Here's how the part is built. I have some questions about the finished solid (model axes, mm). A direction names the side the tool comes from. Round coordinates to 2 decimals unless told otherwise and drop trailing zeros. Loops run counter-clockwise (first coordinate to the right, second up) from the corner with the lowest first, then second, coordinate; pieces in that order, holes last. Notation, with made-up numbers: M 29,-18.5 L 40,-18.5 A5 ccw 40,-13.5 Z; hole C 76.5,37.5 d2. An arc over 180 degrees is marked long. Use a Markdown table: item, result.
from build123d import *

# Parameters (mm, degrees)
F1_DEPTH = 127
F2_DEPTH = 50.8


with BuildPart() as f1:
    # F0 (on Front) → F1 (new body)
    with BuildSketch(Plane.XZ):
        Polygon((-26.435141, -57.215432), (-73.037098, -57.215432), (-73.037098, -75.057486), (73.037098, -75.057486), (73.037098, -57.215432), (1.397706, -57.215432), align=None)
    extrude(amount=F1_DEPTH)

    # F0 (on Front) → F2 (join)
    with BuildSketch(Plane.XZ):
        with BuildLine():
            ThreePointArc((-28.038343, -31.901021), (-31.207175, -44.80968), (-26.435141, -57.215432))
            Line((-26.435141, -57.215432), (1.397706, -57.215432))
            ThreePointArc((1.397706, -57.215432), (8.385599, -39.591583), (13.815437, -21.427125))
            ThreePointArc((13.815437, -21.427125), (14.783315, -18.607969), (15.555009, -15.728923))
            ThreePointArc((15.555009, -15.728923), (16.072278, -13.136524), (16.430436, -10.517398))
            ThreePointArc((16.430436, -10.517398), (15.978576, 1.750902), (12.102647, 13.399617))
            ThreePointArc((12.102647, 13.399617), (10.780812, 17.568694), (10.917028, 21.940181))
            ThreePointArc((10.917028, 21.940181), (14.382768, 26.766265), (15.82858, 32.529256))
            ThreePointArc((15.82858, 32.529256), (15.174964, 38.029758), (12.669052, 42.96971))
            ThreePointArc((12.669052, 42.96971), (-0.488801, 49.284531), (-13.232451, 42.170782))
            ThreePointArc((-13.232451, 42.170782), (-15.565366, 36.45211), (-15.536207, 30.275958))
            ThreePointArc((-15.536207, 30.275958), (-14.031369, 26.055756), (-11.405967, 22.425065))
            ThreePointArc((-11.405967, 22.425065), (-9.956311, 16.857974), (-10.306361, 11.115896))
            ThreePointArc((-10.306361, 11.115896), (-16.642557, 0.773962), (-17.132959, -11.344721))
            ThreePointArc((-17.132959, -11.344721), (-19.235101, -19.303269), (-23.144801, -26.547005))
            ThreePointArc((-23.144801, -26.547005), (-24.70678, -28.600459), (-26.416359, -30.532761))
            ThreePointArc((-26.416359, -30.532761), (-27.040856, -31.171473), (-27.681515, -31.793972))
            ThreePointArc((-27.681515, -31.793972), (-27.875593, -31.795282), (-28.038343, -31.901021))
        make_face()
        with BuildLine():
            ThreePointArc((12.669052, 42.96971), (15.174964, 38.029758), (15.82858, 32.529256))
            ThreePointArc((15.82858, 32.529256), (21.831874, 39.038084), (21.566212, 47.888722))
            Line((21.566212, 47.888722), (12.669052, 42.96971))
        make_face()
        with BuildLine():
            ThreePointArc((-27.039211, 44.109747), (-25.18838, 33.949385), (-15.536207, 30.275958))
            ThreePointArc((-15.536207, 30.275958), (-15.565366, 36.45211), (-13.232451, 42.170782))
            Line((-13.232451, 42.170782), (-27.039211, 44.109747))
        make_face()
        with BuildLine():
            ThreePointArc((-50.62522, 5.92908), (-35.638015, -10.387821), (-26.416359, -30.532761))
            ThreePointArc((-26.416359, -30.532761), (-24.70678, -28.600459), (-23.144801, -26.547005))
            ThreePointArc((-23.144801, -26.547005), (-29.007683, -7.357016), (-44.044595, 5.92908))
            ThreePointArc((-44.044595, 5.92908), (-51.27709, 19.259676), (-49.117848, 34.271386))
            ThreePointArc((-49.117848, 34.271386), (-50.091291, 37.454091), (-52.961979, 35.769943))
            ThreePointArc((-52.961979, 35.769943), (-55.552639, 20.555151), (-50.62522, 5.92908))
        make_face()
    extrude(amount=F2_DEPTH)


solid = f1.part
1. Imagine slicing it at A-A, the plane z = 3.5. Write out the boundary of the cut face in (x, y), then the cut area to 3 significant figures.
Answer sheet:
| item | result |
|---|---|
| outline | M -47.73,-50.8 L -39.75,-50.8 L -39.75,0 L -47.73,0 Z; M -15.63,-50.8 L 15.62,-50.8 L 15.62,0 L -15.63,0 Z |
| area | 1,990 mm2 |
2. We'd pull the mould along X, two halves only. Please class faces 4 (the face through (14.347, -25.044, 26.69)), 5 (the face through (-28.855, -25.044, -7.597)), 6 (the face through (1, -63, -57.215)): +X half, -X half, draft (parallel to the pull), parting line (faces both ways), or undercut.
Answer sheet:
| item | result |
|---|---|
| face 4 | +X half |
| face 5 | undercut |
| face 6 | draft |
3. For pin 1 Ø1 at (x, y) = (40, -35) entering from +Z; pin 2 Ø10 at (y, z) = (-38, -7.5) entering from +X; pin 3 Ø6 at (x, z) = (2, 32) entering from -Y, each with a flat end and sliding along its axis, tell me the tip position at first contact or that it passes through.
Answer sheet:
| item | result |
|---|---|
| pin 1 | z = -57.22 |
| pin 2 | x = 16.67 |
| pin 3 | y = -50.8 |
4. I need wall thicknesses on probe 1 along Z at (x, y) = (41, -91); probe 2 along Y at (x, z) = (-5.5, 4.5); probe 3 along Z at (x, y) = (3.5, -38). Which ranges of each line are inside material? Lowest first, please. Write a range as from..to.
Answer sheet:
| item | result |
|---|---|
| probe 1 | -75.06..-57.22 |
| probe 2 | -50.8..0 |
| probe 3 | -75.06..-57.22, -52.36..48.9 |
5. Imagine slicing it at D-D, the plane y = -88. Write out the boundary of the cut face in (x, z).
Answer sheet:
| item | result |
|---|---|
| outline | M -73.04,-75.06 L 73.04,-75.06 L 73.04,-57.22 L -73.04,-57.22 Z |
6. Which directions (+Z, -Z, +X, -X, +Y, -Y) give clear straight access to the entire face, cutting with the end or side of a thin tool? Please do faces 1 (the face through (-8, -50.8, -3)), 2 (the face through (-51.24, -25.04, 19.05)), 3 (the face through (16.066, -25.044, -13.173)).
Answer sheet:
| item | result |
|---|---|
| face 1 | +Z, +X, -X, -Y |
| face 2 | +Y, -Y |
| face 3 | +X, +Y, -Y |
7. Imagine slicing it at C-C, the plane z = -44. Write out the boundary of the cut face in (x, y), then the cut area to 3 significant figures.
Answer sheet:
| item | result |
|---|---|
| outline | M -31.24,-50.8 L 6.8,-50.8 L 6.8,0 L -31.24,0 Z |
| area | 1,930 mm2 |
